Input: part model. Units: mm. Frame: model coordinates. A direction names the side the tool comes from. Give positions to 0.01 mm unless a question says otherwise; leave off trailing zeros. Loops run counter-clockwise (first coordinate to the right, second up) from the corner with the lowest first, then second, coordinate; pieces in that order, holes last. Notation, with made-up numbers: (83.5, -10.5) - (89.5, -10.5) arc R32 ccw to (89.5, 21.5) - close; hole circle Ø4 at (17.25, -4). An arc over 180 degrees is marked (long way). One line per question, with ' | ' between items. Start each with the question number.
from build123d import *

# Parameters (mm, degrees)
SKETCH1_R               = 50
BOSS_EXTRUDE1_DEPTH     = 140
SKETCH2_W               = 10
SKETCH2_H               = 60
BOSS_EXTRUDE2_START     = 100
SKETCH3_R               = 50
BOSS_EXTRUDE2_DEPTH     = 100
SKETCH4_R               = 169.268161275
BOSS_EXTRUDE3_DEPTH     = 10
FILLET2_R               = 50
CUT_EXTRUDE1_DEPTH      = 278.314660346
CUT_EXTRUDE1_DEPTH_BACK = 278.314660346
SKETCH5_W               = 221.299470988
SKETCH5_H               = 358.524470465


with BuildPart() as part:
    # Sketch1 → Boss-Extrude1 (new body)
    with BuildSketch(Plane(origin=(0, 0, 0), x_dir=(0, 0, -1), z_dir=(1, 0, 0))):
        Circle(SKETCH1_R)
    extrude(amount=BOSS_EXTRUDE1_DEPTH)

    # Sketch2 → Revolve1 (revolve)
    with BuildSketch(Plane(origin=(0, 0, 0), x_dir=(1, 0, 0), z_dir=(0, 1, 0)), mode=Mode.PRIVATE) as revolve1_sk:
        with Locations((15, 30)):
            Rectangle(SKETCH2_W, SKETCH2_H)
        with Locations((125, 30)):
            Rectangle(SKETCH2_W, SKETCH2_H)
    revolve(revolve1_sk.sketch.rotate(Axis((0, 0, 0), (1, 0, 0)), 180), axis=Axis((0, 0, 0), (1, 0, 0)))

    # Sketch3 → Boss-Extrude2 (add)
    with BuildSketch(Plane.ZY.offset(BOSS_EXTRUDE2_START)):
        Circle(SKETCH3_R)
    extrude(amount=-BOSS_EXTRUDE2_DEPTH)

    # Sketch4 → Boss-Extrude3 (add)
    with BuildSketch(Plane.ZY.offset(100)):
        Circle(SKETCH4_R)
    extrude(amount=BOSS_EXTRUDE3_DEPTH)

    # Fillet2
    fillet2_edges = [part.edges().sort_by_distance(p)[0] for p in [
        (-100, 0, -50),
    ]]
    fillet(fillet2_edges, radius=FILLET2_R)

    # Sketch5 → Cut-Extrude1 (cut, two sides: drawn at the far end of the back side and taken through both)
    with BuildSketch(Plane.XY.offset(-CUT_EXTRUDE1_DEPTH_BACK)):
        with Locations((-135.649735494, -5.556646105)):
            Rectangle(SKETCH5_W, SKETCH5_H)
    extrude(amount=CUT_EXTRUDE1_DEPTH + CUT_EXTRUDE1_DEPTH_BACK, mode=Mode.SUBTRACT)

    # Sketch6 → Cut-Revolve1 (revolve, cut)
    with BuildSketch(Plane(origin=(0, 0, 0), x_dir=(1, 0, 0), z_dir=(0, 1, 0)), mode=Mode.PRIVATE) as cut_revolve1_sk:
        Polygon((-37.123590864, 20), (0, 20), (0, 63.419467726), (-45.130639874, 53.302044746), align=None)
    revolve(cut_revolve1_sk.sketch.rotate(Axis((-42.77009101, 0, 0), (1, 0, 0)), 180), axis=Axis((-42.77009101, 0, 0), (1, 0, 0)), mode=Mode.SUBTRACT)


solid = part.part
Q1. Draft query along X for faces 5 (the face through (-25, 0, 0)), 6 (the face through (15.07, -50.59, 32.26)), 7 (the face through (69.3, 15.02, -47.69)), 8 (the face through (140, 1, 1)). Return one class per face: +X half, -X half, draft (parallel to the pull), parting line (faces both ways), or undercut.
Q2. Line query: L1, parallel to X at y = 53.5, z = -13.5; L2, parallel to X at y = -28, z = 26.5; L3, parallel to Y at x = 14, z = 12. Output: solid intervals per line, ascending. Write a range as from..to.
Q3. Access query for faces 1 (the face through (130, -45, 23)), 2 (the face through (125.07, -50.59, 32.26)), 3 (the face through (20, -45, 23)), 4 (the face through (4.93, 15.02, -47.69)). Directions: +Z, -Z, +X, -X, +Y, -Y. A direction counts if a zero-diameter tool reaches every point of the face in a straight line with its end or side. Return the directions, or none.
Q4. Section A-A, the plane z = -48. Output: boundary loops of the cut face in (x, y), plus the area to 3 significant figures.
Q5. First-contact query: pin 1 (10 mm diameter, centred on x = 63.5, z = -35, fed in from -Y); pin 2 (12 mm diameter, centred on x = 31, z = 39.5, fed in from +Y); pin 3 (8 mm diameter, centred on x = 54, y = -5, fed in from -Z). Flat tips, straight axial feed; report the tip coordinate or a pass-through.
Q6. Section B-B, the plane y = 0. Output: boundary loops of the cut face in (x, z).
Q7. Section C-C, the plane x = 27.5. Output: boundary loops of the cut face in (y, z), plus the area to 3 significant figures.
Solved:
1) face 5: -X half | face 6: draft | face 7: undercut | face 8: +X half
2) L1: x = 10..20, 120..130 | L2: x = 0..140 | L3: y = -58.79..58.79
3) face 1: +X | face 2: +X, -X | face 3: none | face 4: -X
4) outline: (0, -14) - (10, -14) - (10, -36) - (20, -36) - (20, -14) - (120, -14) - (120, -36) - (130, -36) - (130, -14) - (140, -14) - (140, 14) - (130, 14) - (130, 36) - (120, 36) - (120, 14) - (20, 14) - (20, 36) - (10, 36) - (10, 14) - (0, 14) - close | area: 4,800 mm²
5) pin 1: stops at y = -40 | pin 2: stops at y = 37.12 | pin 3: stops at z = -49.99
6) outline: (-25, -20) - (0, -20) - (0, -50) - (10, -50) - (10, -60) - (20, -60) - (20, -50) - (120, -50) - (120, -60) - (130, -60) - (130, -50) - (140, -50) - (140, 50) - (130, 50) - (130, 60) - (120, 60) - (120, 50) - (20, 50) - (20, 60) - (10, 60) - (10, 50) - (0, 50) - (0, 20) - (-25, 20) - close
7) outline: circle Ø100 at (0, 0) | area: 7,850 mm²
